from build123d import *

# Parameters (mm, degrees)
F1_DEPTH = 917.5
F2_DEPTH = 40
F3_W     = 199
F3_H     = 770.7896669658
F4_DEPTH = 13
F5_DEPTH = 110


with BuildPart() as f1:
    # F0 (on Front) → F1 (new body)
    with BuildSketch(Plane.XZ):
        with BuildLine():
            ThreePointArc((-102.5, -13.5), (-101.767766953, -15.267766953), (-100, -16))
            Line((-100, -16), (100, -16))
            ThreePointArc((100, -16), (101.767766953, -15.267766953), (102.5, -13.5))
            Line((102.5, -13.5), (102.5, 0))
            Line((102.5, 0), (99.5, 0))
            Line((99.5, 0), (99.5, -10.5))
            ThreePointArc((99.5, -10.5), (98.767766953, -12.267766953), (97, -13))
            Line((97, -13), (-97, -13))
            ThreePointArc((-97, -13), (-98.767766953, -12.267766953), (-99.5, -10.5))
            Line((-99.5, -10.5), (-99.5, 0))
            Line((-99.5, 0), (-102.5, 0))
            Line((-102.5, 0), (-102.5, -13.5))
        make_face()
        with BuildLine():
            Line((-96.5, 0), (-99.5, 0))
            Line((-99.5, 0), (-99.5, -10.5))
            ThreePointArc((-99.5, -10.5), (-98.767766953, -12.267766953), (-97, -13))
            Line((-97, -13), (97, -13))
            ThreePointArc((97, -13), (98.767766953, -12.267766953), (99.5, -10.5))
            Line((99.5, -10.5), (99.5, 0))
            Line((99.5, 0), (96.5, 0))
            Line((96.5, 0), (96.5, -7.5))
            ThreePointArc((96.5, -7.5), (95.767766953, -9.267766953), (94, -10))
            Line((94, -10), (-94, -10))
            ThreePointArc((-94, -10), (-95.767766953, -9.267766953), (-96.5, -7.5))
            Line((-96.5, -7.5), (-96.5, 0))
        make_face()
    extrude(amount=F1_DEPTH)

    # F0 (on Front) → F2 (cut)
    with BuildSketch(Plane.XZ):
        with BuildLine():
            ThreePointArc((-102.5, -13.5), (-101.767766953, -15.267766953), (-100, -16))
            Line((-100, -16), (100, -16))
            ThreePointArc((100, -16), (101.767766953, -15.267766953), (102.5, -13.5))
            Line((102.5, -13.5), (102.5, 0))
            Line((102.5, 0), (99.5, 0))
            Line((99.5, 0), (99.5, -10.5))
            ThreePointArc((99.5, -10.5), (98.767766953, -12.267766953), (97, -13))
            Line((97, -13), (-97, -13))
            ThreePointArc((-97, -13), (-98.767766953, -12.267766953), (-99.5, -10.5))
            Line((-99.5, -10.5), (-99.5, 0))
            Line((-99.5, 0), (-102.5, 0))
            Line((-102.5, 0), (-102.5, -13.5))
        make_face()
    extrude(amount=F2_DEPTH, mode=Mode.SUBTRACT)

    # F3 (on face) → F4 (cut)
    with BuildSketch(Plane.XY):
        with Locations((0, -428.3948334829)):
            Rectangle(F3_W, F3_H)
    extrude(amount=-F4_DEPTH, mode=Mode.SUBTRACT)

    # F5 (cut): a face of the model
    f5_faces = [f1.faces().sort_by_distance(p)[0] for p in [
        (0, -813.7896669658, -10.9004362027),
    ]]
    extrude(f5_faces, amount=-F5_DEPTH, mode=Mode.SUBTRACT)


solid = f1.part
Model file for the job. Use its own axes, mm. A direction names the side the tool comes from. Give positions to 0.01 mm unless a question says otherwise; leave off trailing zeros. Order: outer loops, then holes, each group sorted by start corner. A loop starts at its lowest first (then second) coordinate and runs counter-clockwise, first axis right, second up. Notation, with made-up numbers: M 62.25,-12.75 L 99.25,-12.75 A11 ccw 99.25,7.25 Z; hole C 15,66 d1. An arc over 180 degrees is marked long. Put each result on its own line as item: value. Start each with the question number.
(1) Band-saw the part on A-A on z = -4.5. Give the cut face in (x, y), then the cut area to 3 significant figures.
(2) Band-saw the part on B-B on y = -313. Give the cut face in (x, z), then the cut area to 3 significant figures.
(3) Tool access for faces 1 (the face through (1, -21, -10)), 2 (the face through (0, -917.5, -14)): list every direction of +Z, -Z, +X, -X, +Y, -Y with a clear straight run to the whole face (end or side of a thin tool).
(4) Pull direction X, two halves, no side cores. Call faces 3 (the face through (1, -20, -13)), 4 (the face through (-1, -474, -13)): released by +X, released by -X, zero draft, split by the parting line, or undercut.
(5) Pin check, flat tips, straight feed: pin 1 Ø4 at (y, z) = (-30.5, -3) entering from +X; pin 2 Ø1.5 at (x, z) = (55, -11) entering from +Y; pin 3 Ø10 at (x, y) = (40.5, -596.5) entering from +Z; pin 4 Ø21.5 at (x, y) = (3, -11) entering from +Z. Stop position of each tip, or through.
(6) Band-saw the part on C-C on x = 36. Give the cut face in (y, z), then the cut area to 3 significant figures.
(7) Drill centre lines: L1, parallel to X at y = -284, z = -1; L2, parallel to Z at x = -47.5, y = -506.5; L3, parallel to Y at x = 48, z = -14.5. Where is each one in solid material? Low to high. Write a range as [from, to].
Results below:
1. outline: M -102.5,-917.5 L -99.5,-917.5 L -99.5,-43 L -96.5,-43 L -96.5,0 L -99.5,0 L -99.5,-40 L -102.5,-40 Z; M 96.5,-43 L 99.5,-43 L 99.5,-917.5 L 102.5,-917.5 L 102.5,-40 L 99.5,-40 L 99.5,0 L 96.5,0 Z
1. area: 5,520 mm2
2. outline: M -102.5,-13.5 A2.5 ccw -100,-16 L 100,-16 A2.5 ccw 102.5,-13.5 L 102.5,0 L 99.5,0 L 99.5,-13 L -99.5,-13 L -99.5,0 L -102.5,0 Z
2. area: 690 mm2
3. face 1: +Z, +Y, -Y
3. face 2: +Z, -Z, +X, -X, -Y
4. face 3: zero draft
4. face 4: undercut
5. pin 1: stops at x = 99.5
5. pin 2: stops at y = 0
5. pin 3: stops at z = -13
5. pin 4: stops at z = -10
6. outline: M -917.5,-16 L -40,-16 L -40,-13 L 0,-13 L 0,-10 L -43,-10 L -43,-13 L -917.5,-13 Z
6. area: 2,760 mm2
7. L1: x = [-102.5, -99.5], [99.5, 102.5]
7. L2: z = [-16, -13]
7. L3: y = [-917.5, -40]
